```python
from build123d import *

# Parameters (mm, degrees)
EXTRUDE_1_DEPTH = 100


with BuildPart() as part:
    # 草图1 → 凸台-拉伸1 (new body)
    with BuildSketch(Plane.XY):
        with BuildLine():
            Line((0, -1.3), (0, 0))
            Line((0, 0), (0.876117478, 0))
            ThreePointArc((0.876117478, 0), (1.025270289, -0.066757968), (1.074851714, -0.222465609))
            Line((1.074851714, -0.222465609), (0.762425857, -2.986232805))
            Line((0.762425857, -2.986232805), (1.55, -4.165282478))
            Line((1.55, -4.165282478), (1.134225832, -4.443008676))
            Line((1.134225832, -4.443008676), (0.675396165, -3.756110847))
            Line((0.675396165, -3.756110847), (0.45, -5.75))
            Line((0.45, -5.75), (0.45, -10.55))
            ThreePointArc((0.45, -10.55), (0.508578644, -10.691421356), (0.65, -10.75))
            Line((0.65, -10.75), (6.95, -10.75))
            ThreePointArc((6.95, -10.75), (7.091421356, -10.691421356), (7.15, -10.55))
            Line((7.15, -10.55), (7.15, -5.75))
            Line((7.15, -5.75), (6.924603835, -3.756110847))
            Line((6.924603835, -3.756110847), (6.465774168, -4.443008676))
            Line((6.465774168, -4.443008676), (6.05, -4.165282478))
            Line((6.05, -4.165282478), (6.837574143, -2.986232805))
            Line((6.837574143, -2.986232805), (6.525148286, -0.222465609))
            ThreePointArc((6.525148286, -0.222465609), (6.574729711, -0.066757968), (6.723882522, 0))
            Line((6.723882522, 0), (7.6, 0))
            Line((7.6, 0), (7.6, -1.3))
            Line((7.6, -1.3), (7.30173337, -1.3))
            Line((7.30173337, -1.3), (7.9, -5.707743265))
            Line((7.9, -5.707743265), (7.9, -11))
            ThreePointArc((7.9, -11), (7.753553391, -11.353553391), (7.4, -11.5))
            Line((7.4, -11.5), (0.2, -11.5))
            ThreePointArc((0.2, -11.5), (-0.153553391, -11.353553391), (-0.3, -11))
            Line((-0.3, -11), (-0.3, -5.707743265))
            Line((-0.3, -5.707743265), (0.29826663, -1.3))
            Line((0.29826663, -1.3), (0, -1.3))
        make_face()
    extrude(amount=EXTRUDE_1_DEPTH)


solid = part.part
```
Read the model definition and answer for the solid it produces. Units are mm, in the model's axes. A direction names the side the tool comes from. Round coordinates to 2 decimals unless told otherwise and drop trailing zeros. Loops run counter-clockwise (first coordinate to the right, second up) from the corner with the lowest first, then second, coordinate; pieces in that order, holes last. Notation, with made-up numbers: (86, 30) -> (106, 30) arc R11 cw to (106, 50) -> close; hole circle Ø9 at (84.25, 85). An arc over 180 degrees is marked (long way). One line per item, written item: value.
1) For faces 1 (the face through (0.45, -8, 49)), 2 (the face through (0, -3.5, 49.3)), 3 (the face through (7.6, -3.5, 49.3)), determine the directions among +Z, -Z, +X, -X, +Y, -Y from which every point of the face is accessible in a straight line to the end or side of a thin tool.
Answer list:
face 1: +Z, -Z
face 2: +Z, -Z, -X
face 3: +Z, -Z, +X
2) Flat-ended cylindrical pins translate along their axes: P1, Ø1, axis at y = -0.5, z = 71.5, coming from the +X side; P2, Ø0.6, axis at y = -0.5, z = 68, coming from the -X side. Find the tip coordinate at first contact, or state that the pin passes through.
Answer list:
P1: stops at x = 7.6
P2: stops at x = 0
3) Consider L1, parallel to X at y = -6.25, z = 90; L2, parallel to Y at x = 3.75, z = 50. Determine where each line is inside the solid, lowest interval first. Write a range as [from, to].
Answer list:
L1: x = [-0.3, 0.45], [7.15, 7.9]
L2: y = [-11.5, -10.75]
4) A cutting plane is placed at A-A (y = -7.5). Determine the outline of the cut face in (x, z).
Answer list:
outline: (-0.3, 0) -> (0.45, 0) -> (0.45, 100) -> (-0.3, 100) -> close; (7.15, 0) -> (7.9, 0) -> (7.9, 100) -> (7.15, 100) -> close
5) The mould has two halves that part along Y. Classify faces 4 (the face through (7.9, -8, 49)), 5 (the face through (4, -11.5, 49)), 6 (the face through (0.92, -1.59, 49.3)): pulls with the +Y half, pulls with the -Y half, needs draft (parallel to the pull), parting line crosses it, or undercut.
Answer list:
face 4: needs draft
face 5: pulls with the -Y half
face 6: undercut
6) A cutting plane is placed at C-C (x = 3.5). Determine the outline of the cut face in (y, z).
Answer list:
outline: (-11.5, 0) -> (-10.75, 0) -> (-10.75, 100) -> (-11.5, 100) -> close
